```python
from build123d import *

# Parameters (mm, degrees)
ENL_V_MAT_EXTRU_2_DEPTH = 9
CHANFREIN1_SIZE         = 0.25
CONG_1_R                = 0.5
ESQUISSE4_R             = 10
ENL_V_MAT_EXTRU_3_DEPTH = 23
CONG_2_R                = 1
ESQUISSE5_W             = 75.40554743
ESQUISSE5_H             = 27.453522384
ENL_V_MAT_EXTRU_4_DEPTH = 30
COQUE1_START            = -43
COQUE1_DEPTH            = 42
COQUE1_START_2          = -36
COQUE1_2_DEPTH          = 28
COQUE1_START_3          = -48
COQUE1_3_DEPTH          = 5
COQUE1_4_DEPTH          = 4.5
COQUE1_START_4          = -5.5
COQUE1_5_DEPTH          = 4.5
COQUE1_START_5          = -1
COQUE1_6_DEPTH          = 8.25
COQUE1_START_6          = -43.25
COQUE1_7_DEPTH          = 0.25
COQUE1_START_7          = 7.25
COQUE1_8_DEPTH          = 3
COQUE1_9_DEPTH          = 2.25
COQUE1_10_DEPTH         = 0.25
ENL_V_START             = -10
ENL_V_MAT_EXTRU_5_DEPTH = 10
BOSS_EXTRU_1_REACH      = 58.577
BOSS_EXTRU_1_END_RADIUS = 7.5
ESQUISSE7_R             = 2.5
ESQUISSE9_R             = 2.25
ENL_V_MAT_EXTRU_6_DEPTH = 7
D_GAGEMENT_M22_D        = 2.4
BOSS_EXTRU_2_START      = 1
ESQUISSE11_R            = 2.5
ESQUISSE11_R_2          = 1.5
BOSS_EXTRU_2_DEPTH      = 1
ESQUISSE12_R            = 1.5
ESQUISSE12_R_2          = 1.2
ENL_V_MAT_EXTRU_7_DEPTH = 1


# Read off the part's stored shape, not the designer's step: Coque1
with BuildPart() as part:
    # Esquisse1 → Révolution1 (revolve)
    with BuildSketch(Plane(origin=(0, 0, 0), x_dir=(1, 0, 0), z_dir=(0, 1, 0))):
        Polygon((20, 0), (4, 0), (4, -0.25), (3, -0.25), (3, -8.25), (2.5, -8.25), (2.5, -9.25), (3, -9.25), (3, -11.25), (0, -11.25), (0, 49), (8.5, 49), (8.5, 44.25), (10, 44.25), (10, 44), (20, 44), (20, 37.5), (19.5, 37.5), (19.5, 37), (20, 37), (20, 7), (19.5, 7), (19.5, 6.5), (20, 6.5), align=None)
    revolve(axis=Axis((0, 0, 0), (0, 0, -1)))

    # Esquisse3 → Enlèv. mat.-Extru.2 (cut)
    with BuildSketch(Plane.XY.offset(11.25)):
        with BuildLine():
            Line((-2.236067977, 2), (2.236067977, 2))
            ThreePointArc((2.236067977, 2), (0, 3), (-2.236067977, 2))
        make_face()
    extrude(amount=-ENL_V_MAT_EXTRU_2_DEPTH, mode=Mode.SUBTRACT)

    # Chanfrein1
    chanfrein1_edges = [part.edges().sort_by_distance(p)[0] for p in [
        (0, -3, 11.25),
    ]]
    chamfer(chanfrein1_edges, length=CHANFREIN1_SIZE)

    # Congé1
    cong_1_edges = [part.edges().sort_by_distance(p)[0] for p in [
        (-20, 0, 0),
        (-20, 0, -44),
    ]]
    fillet(cong_1_edges, radius=CONG_1_R)

    # Esquisse4 → Enlèv. mat.-Extru.3 (cut)
    with BuildSketch(Plane(origin=(0, -29, 0), x_dir=(-1, 0, 0), z_dir=(0, 1, 0))):
        with Locations(Location((0, -22, 0), (0, 0, 270))):
            Circle(ESQUISSE4_R)
    extrude(amount=ENL_V_MAT_EXTRU_3_DEPTH, mode=Mode.SUBTRACT)

    # Congé2
    cong_2_edges = [part.edges().sort_by_distance(p)[0] for p in [
        (-0.062948247, -19.999900935, -12.000198118),
    ]]
    fillet(cong_2_edges, radius=CONG_2_R - 0.0001)  # a hair under: the kernel refuses the full size

    # Esquisse5 → Enlèv. mat.-Extru.4 (cut, symmetric)
    with BuildSketch(Plane(origin=(0, 0, 0), x_dir=(0, 0, -1), z_dir=(1, 0, 0))):
        with Locations((20.552947191, -13.726761192)):
            Rectangle(ESQUISSE5_W, ESQUISSE5_H)
    extrude(amount=ENL_V_MAT_EXTRU_4_DEPTH, both=True, mode=Mode.SUBTRACT)

    # Coque1 outline → Coque1 (cut)
    with BuildSketch(Plane.XY.offset(COQUE1_START)):
        with BuildLine():
            ThreePointArc((18.5, 0), (0, 18.5), (-18.5, 0))
            Line((-18.5, 0), (18.5, 0))
        make_face()
    extrude(amount=COQUE1_DEPTH, mode=Mode.SUBTRACT)

    # Coque1 2 outline → Coque1 2 (cut)
    with BuildSketch(Plane.XY.offset(COQUE1_START_2)):
        with BuildLine():
            Line((-19, 0), (-18.5, 0))
            ThreePointArc((-18.5, 0), (0, 18.5), (18.5, 0))
            Line((18.5, 0), (19, 0))
            ThreePointArc((19, 0), (0, 19), (-19, 0))
        make_face()
    extrude(amount=COQUE1_2_DEPTH, mode=Mode.SUBTRACT)

    # Coque1 3 outline → Coque1 3 (cut)
    with BuildSketch(Plane.XY.offset(COQUE1_START_3)):
        with BuildLine():
            ThreePointArc((7.5, 0), (0, 7.5), (-7.5, 0))
            Line((-7.5, 0), (7.5, 0))
        make_face()
    extrude(amount=COQUE1_3_DEPTH, mode=Mode.SUBTRACT)

    # Coque1 4 outline → Coque1 4 (cut)
    with BuildSketch(Plane.XY.offset(COQUE1_START)):
        with BuildLine():
            Line((-19, 0), (-18.5, 0))
            ThreePointArc((-18.5, 0), (0, 18.5), (18.5, 0))
            Line((18.5, 0), (19, 0))
            ThreePointArc((19, 0), (0, 19), (-19, 0))
        make_face()
    extrude(amount=COQUE1_4_DEPTH, mode=Mode.SUBTRACT)

    # Coque1 5 outline → Coque1 5 (cut)
    with BuildSketch(Plane.XY.offset(COQUE1_START_4)):
        with BuildLine():
            Line((-19, 0), (-18.5, 0))
            ThreePointArc((-18.5, 0), (0, 18.5), (18.5, 0))
            Line((18.5, 0), (19, 0))
            ThreePointArc((19, 0), (0, 19), (-19, 0))
        make_face()
    extrude(amount=COQUE1_5_DEPTH, mode=Mode.SUBTRACT)

    # Coque1 6 outline → Coque1 6 (cut)
    with BuildSketch(Plane.XY.offset(COQUE1_START_5)):
        with BuildLine():
            ThreePointArc((-1.732050808, 1), (-1.931851653, 0.51763809), (-2, 0))
            Line((-2, 0), (2, 0))
            ThreePointArc((2, 0), (1.931851653, 0.51763809), (1.732050808, 1))
            Line((1.732050808, 1), (-1.732050808, 1))
        make_face()
    extrude(amount=COQUE1_6_DEPTH, mode=Mode.SUBTRACT)

    # Coque1 7 outline → Coque1 7 (cut)
    with BuildSketch(Plane.XY.offset(COQUE1_START_6)):
        with BuildLine():
            Line((-9, 0), (-7.5, 0))
            ThreePointArc((-7.5, 0), (0, 7.5), (7.5, 0))
            Line((7.5, 0), (9, 0))
            ThreePointArc((9, 0), (0, 9), (-9, 0))
        make_face()
    extrude(amount=COQUE1_7_DEPTH, mode=Mode.SUBTRACT)

    # Coque1 8 outline → Coque1 8 (cut)
    with BuildSketch(Plane.XY.offset(COQUE1_START_7)):
        with BuildLine():
            Line((1.118033989, 1), (-1.118033989, 1))
            ThreePointArc((-1.118033989, 1), (-1.401258538, 0.535233134), (-1.5, 0))
            Line((-1.5, 0), (1.5, 0))
            ThreePointArc((1.5, 0), (1.401258538, 0.535233134), (1.118033989, 1))
        make_face()
    extrude(amount=COQUE1_8_DEPTH, mode=Mode.SUBTRACT)

    # Coque1 9 outline → Coque1 9 (cut)
    with BuildSketch(Plane.XY.offset(COQUE1_START_5)):
        with BuildLine():
            Line((-1.732050808, 1), (1.732050808, 1))
            ThreePointArc((1.732050808, 1), (0, 2), (-1.732050808, 1))
        make_face()
    extrude(amount=COQUE1_9_DEPTH, mode=Mode.SUBTRACT)

    # Coque1 10 outline → Coque1 10 (cut)
    with BuildSketch(Plane.XY.offset(COQUE1_START_5)):
        with BuildLine():
            ThreePointArc((-2, 0), (0, 2), (2, 0))
            Line((2, 0), (3, 0))
            ThreePointArc((3, 0), (0, 3), (-3, 0))
            Line((-3, 0), (-2, 0))
        make_face()
    extrude(amount=COQUE1_10_DEPTH, mode=Mode.SUBTRACT)

    # Esquisse6 → Enlèv. mat.-Extru.5 (cut)
    with BuildSketch(Plane.XY.offset(-48).offset(ENL_V_START)):
        with BuildLine():
            Line((-7.5, 0), (7.5, 0))
            ThreePointArc((7.5, 0), (0, 7.5), (-7.5, 0))
        make_face()
    extrude(amount=ENL_V_MAT_EXTRU_5_DEPTH, mode=Mode.SUBTRACT)

    # Boss.-Extru.1: up to this cylinder (the profile starts inside it)
    boss_extru_1_end = Plane(origin=(0, 0, -46.5), z_dir=(0, 0, 1)) * Cylinder(BOSS_EXTRU_1_END_RADIUS, 133.154, mode=Mode.PRIVATE)
    # Esquisse7 → Boss.-Extru.1 (add, up to the surface)
    with BuildSketch(Plane(origin=(0, 0, 0), x_dir=(1, 0, 0), z_dir=(0, 1, 0)), mode=Mode.PRIVATE) as boss_extru_1_sk1:
        with Locations(Location((1.5, 46.5, 0), (0, 0, 90))):
            Circle(ESQUISSE7_R)
    boss_extru_1_tool1 = extrude(boss_extru_1_sk1.sketch, amount=BOSS_EXTRU_1_REACH, mode=Mode.PRIVATE) & boss_extru_1_end
    add(boss_extru_1_tool1.solids().sort_by_distance((1.5, 0, -46.5))[0])

    # Esquisse9 → Enlèv. mat.-Extru.6 (cut)
    with BuildSketch(Plane.XZ.offset(-11)):
        with Locations(Location((1.5, -46.5, 0), (0, 0, 90))):
            Circle(ESQUISSE9_R)
    extrude(amount=ENL_V_MAT_EXTRU_6_DEPTH, mode=Mode.SUBTRACT)

    # Dégagement M22 (through all)
    with Locations(Plane(origin=(1.5, 0, -46.5), x_dir=(0, 0, -1), z_dir=(0, -1, 0))):
        with Locations((0, 0)):
            Hole(D_GAGEMENT_M22_D / 2)

    # Esquisse11 → Boss.-Extru.2 (add)
    with BuildSketch(Plane.XZ.offset(BOSS_EXTRU_2_START)):
        with Locations(Location((1.5, -46.5, 0), (0, 0, 270))):
            Circle(ESQUISSE11_R)
        with Locations(Location((1.5, -46.5, 0), (0, 0, 270))):
            Circle(ESQUISSE11_R_2, mode=Mode.SUBTRACT)
    extrude(amount=-BOSS_EXTRU_2_DEPTH)

    # Esquisse12 → Enlèv. mat.-Extru.7 (cut)
    with BuildSketch(Plane.XZ):
        with Locations(Location((1.5, -46.5, 0), (0, 0, 270))):
            Circle(ESQUISSE12_R)
        with Locations(Location((1.5, -46.5, 0), (0, 0, 270))):
            Circle(ESQUISSE12_R_2, mode=Mode.SUBTRACT)
    extrude(amount=-ENL_V_MAT_EXTRU_7_DEPTH, mode=Mode.SUBTRACT)


solid = part.part
```
Source: CAD feature listing. Evaluate the final solid. Frame: model axes, mm. A direction names the side the tool comes from. Round coordinates to 2 decimals unless told otherwise and drop trailing zeros. Loops run counter-clockwise (first coordinate to the right, second up) from the corner with the lowest first, then second, coordinate; pieces in that order, holes last. Notation, with made-up numbers: M -33,75.25 L 6,75.25 A20 ccw 6,107.25 Z; hole C 27,-14.5 d6. An arc over 180 degrees is marked long. Put each result on its own line as item: value.
(1) Access query for faces 4 (the face through (1.6, 19.6, -37)), 5 (the face through (-2.808, 1.056, 10.137)), 6 (the face through (-2.6, 1, 8.25)), 7 (the face through (0, 3, 2)), 8 (the face through (-0.1, 18.7, -5.5)). Directions: +Z, -Z, +X, -X, +Y, -Y. A direction counts if a zero-diameter tool reaches every point of the face in a straight line with its end or side. Return the directions, or none.
Solutions:
face 4: +Y
face 5: +Z, -X, +Y
face 6: -X, +Y
face 7: +Z, +Y
face 8: -Y
(2) Pull-direction query (Z, two-part tool) for faces 1 (the face through (0, 20, -3)), 2 (the face through (0, 12, -44)), 3 (the face through (0, 8, -1)); classes: released by +Z, released by -Z, zero draft, split by the parting line, or undercut.
Solutions:
face 1: zero draft
face 2: released by -Z
face 3: undercut
(3) Section A-A, the plane z = -46.5. Return loops of the section in (x, y).
Solutions:
outline: M -8.5,0 L -7.5,0 A7.5 cw -1,7.43 L -1,-1 L 0,-1 L 0,1 L 0.3,1 L 0.3,4 L -0.75,4 L -0.75,8.47 A8.5 ccw Z; M 2.7,1 L 3,1 L 3,-1 L 4,-1 L 4,6.34 A7.5 cw 7.5,0 L 8.5,0 A8.5 ccw 3.75,7.63 L 3.75,4 L 2.7,4 Z
(4) Section B-B, the plane z = -30. Return loops of the section in (x, y).
Solutions:
outline: M -20,0 L -19,0 A19 cw 19,0 L 20,0 A20 ccw Z
(5) Ray query, line 1 (Z direction, x = 1.5, y = 6.6); line 2 (Z direction, x = -3.5, y = 9.25); line 3 (Z direction, x = -4, y = 16). Return the intervals inside material, ascending. Write a range as [from, to].
Solutions:
line 1: [-49, -48.75], [-44.25, -44], [-1, 0]
line 2: [-44.25, -43], [-1, 0]
line 3: [-44, -43], [-1, 0]
(6) First-contact query: pin 1 (6 mm diameter, centred on x = 11.5, y = 6.5, fed in from -Z); pin 2 (1 mm diameter, centred on x = 2.5, z = -6.5, fed in from +Y); pin 3 (3.5 mm diameter, centred on x = 1.5, z = -46.5, fed in from +Y). Flat tips, straight axial feed; report the tip coordinate or a pass-through.
Solutions:
pin 1: z = -44
pin 2: y = 19.9
pin 3: y = 4
